Check sheet for the modelled part. Datum: model origin and axes. Units: mm. Give positions to 0.01 mm unless a question says otherwise; leave off trailing zeros. Loops run counter-clockwise (first coordinate to the right, second up) from the corner with the lowest first, then second, coordinate; pieces in that order, holes last. Notation, with made-up numbers: (-35, -9.5) - (-17, -9.5) arc R22 cw to (-17, 15.5) - close; hole circle Ø8 at (29.5, 31). An arc over 180 degrees is marked (long way). Answer in a Markdown table with one row per item. Add a question column.
(1) Go/stop test with a flat-tipped pin: P1, Ø9, axis at x = 47.625, z = 355.6, coming from the +Y side. Record where the tip stops, or that it passes through.
(2) Thickness scan on L1, parallel to Z at x = 545.5, y = -0.55; L2, parallel to X at y = -0.3, z = 355.6; L3, parallel to X at y = -0.5, z = 457.2. Record the ranges inside material, lowest first.
(3) Sectioned sample at A-A on z = 558.8. Enter the section's corners in (x, y), then the cut area to 3 significant figures.
from build123d import *

# Parameters (mm, degrees)
F0_W     = 609.6
F0_H     = 609.6
F1_DEPTH = 0.79375
F2_R     = 5.55625
F3_DEPTH = 25.4
F4_R     = 7.14375
F5_DEPTH = 25.4


with BuildPart() as f1:
    # F0 (on Front) → F1 (new body)
    with BuildSketch(Plane.XZ):
        with Locations((304.8, 304.8)):
            Rectangle(F0_W, F0_H)
    extrude(amount=F1_DEPTH)

    # F2 (on face) → F3 (cut)
    with BuildSketch(Plane.XZ.offset(0.79375)):
        with Locations((47.625, 355.6)):
            Circle(F2_R)
        with Locations((47.625, 152.4)):
            Circle(F2_R)
        with Locations((541.3375, 254)):
            Circle(F2_R)
        with Locations((541.3375, 457.2)):
            Circle(F2_R)
    extrude(amount=-F3_DEPTH, mode=Mode.SUBTRACT)

    # F4 (on face) → F5 (cut)
    with BuildSketch(Plane.XZ.offset(0.79375)):
        with Locations((555.625, 558.8)):
            Circle(F4_R)
    extrude(amount=-F5_DEPTH, mode=Mode.SUBTRACT)


solid = f1.part
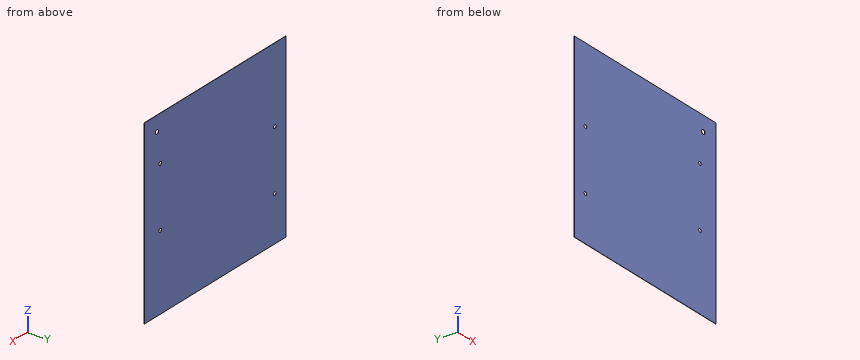
Reply:
| question | item | result |
|---|---|---|
| 1 | P1 | through |
| 2 | L1 | 0 to 250.32, 257.68 to 453.52, 460.88 to 609.6 |
| 2 | L2 | 0 to 42.07, 53.18 to 609.6 |
| 2 | L3 | 0 to 535.78, 546.89 to 609.6 |
| 3 | outline | (0, -0.79) - (548.48, -0.79) - (548.48, 0) - (0, 0) - close; (562.77, -0.79) - (609.6, -0.79) - (609.6, 0) - (562.77, 0) - close |
| 3 | area | 473 mm^2 |
